Can you work these out from the drawing? Everything is in mm from the part's minimum corner. A direction names the side the tool comes from. Coordinates: 2 decimals unless noted, no trailing zeros. Order: outer loops, then holes, each group sorted by start corner. A loop starts at its lowest first (then second) coordinate and runs counter-clockwise, first axis right, second up. Notation, with made-up numbers: (49, 52) -> (68, 52) arc R18 cw to (68, 62) -> close; hole circle Ø8 at (-16.5, 41). An arc over 180 degrees is marked (long way). Write item = value, one per line. Start each with the question number.
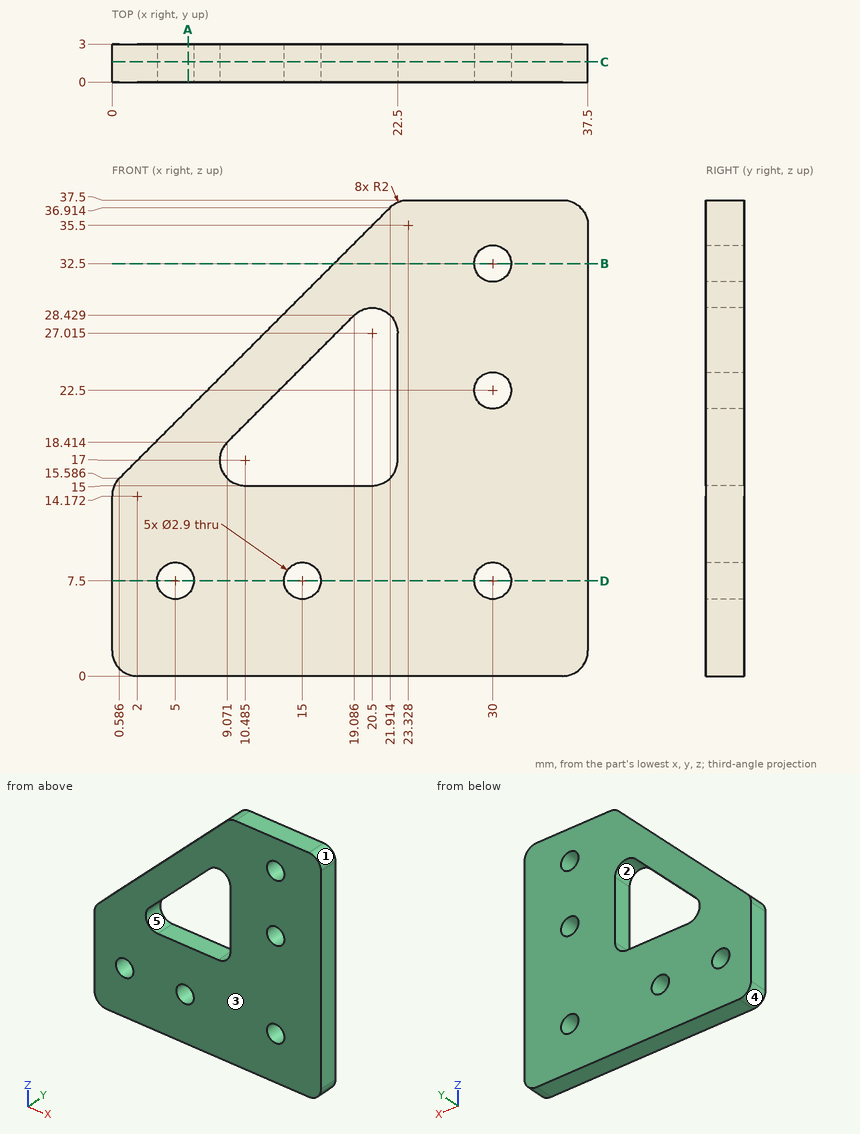
(1) Imagine slicing it at B-B (z = 32.5). Write out the boundary of the cut face in (x, y).
(2) Thinking about a two-plate mould opening in X: for the marked faces 1, 2 and 3, which applies, +X half, -X half, draft (parallel to the pull), parting line (faces both ways), or undercut?
(3) Imagine slicing it at C-C (y = 1.6). Count the separate pieces of the cut face and the enclosed holes in it, plus the area to 3 significant figures.
(4) If I drill on L1, parallel to X at y = 0.7, z = 7.5; L2, parallel to X at y = 2.3, z = 17 (1 decimal); L3, parallel to X at y = 2.45, z = 25.5 (1 decimal), over which ranges is the centre line in solid material (lowest first)? Write a range as from..to.
(5) For P1, Ø1.7, axis at x = 30, z = 32.5, coming from the -Y side; P2, Ø1, axis at y = 2.5, z = 26, coming from the -X side, each with a flat end and sliding along its axis, tell me the tip position at first contact or that it passes through.
(6) Imagine slicing it at A-A (x = 6). Write out the boundary of the cut face in (y, z), plus the area to 3 significant figures.
(7) For the marked faces 4 and 5, which set-ups out of +Z, -Z, +X, -X, +Y, -Y let a thin tool reach every point of the face, with its end or its side?
(8) Imagine slicing it at D-D (z = 7.5). Write out the boundary of the cut face in (x, y).
Result set:
q1.outline = (17.5, 0) -> (28.55, 0) -> (28.55, 3) -> (17.5, 3) -> close; (31.45, 0) -> (37.5, 0) -> (37.5, 3) -> (31.45, 3) -> close
q2.face_1 = +X half
q2.face_2 = undercut
q2.face_3 = draft
q3.separate_pieces = 1
q3.enclosed_holes = 6
q3.area = 986 mm2
q4.L1 = 0..3.55, 6.45..13.55, 16.45..28.55, 31.45..37.5
q4.L2 = 2..8.5, 22.5..37.5
q4.L3 = 10.5..16.2, 22.5..37.5
q5.P1 = through
q5.P2 = 10.5
q6.outline = (0, 0) -> (3, 0) -> (3, 6.45) -> (0, 6.45) -> close; (0, 8.55) -> (3, 8.55) -> (3, 21) -> (0, 21) -> close
q6.area = 56.7 mm2
q7.face_4 = -Z, -X, +Y, -Y
q7.face_5 = +Y, -Y
q8.outline = (0, 0) -> (3.55, 0) -> (3.55, 3) -> (0, 3) -> close; (6.45, 0) -> (13.55, 0) -> (13.55, 3) -> (6.45, 3) -> close; (16.45, 0) -> (28.55, 0) -> (28.55, 3) -> (16.45, 3) -> close; (31.45, 0) -> (37.5, 0) -> (37.5, 3) -> (31.45, 3) -> close
